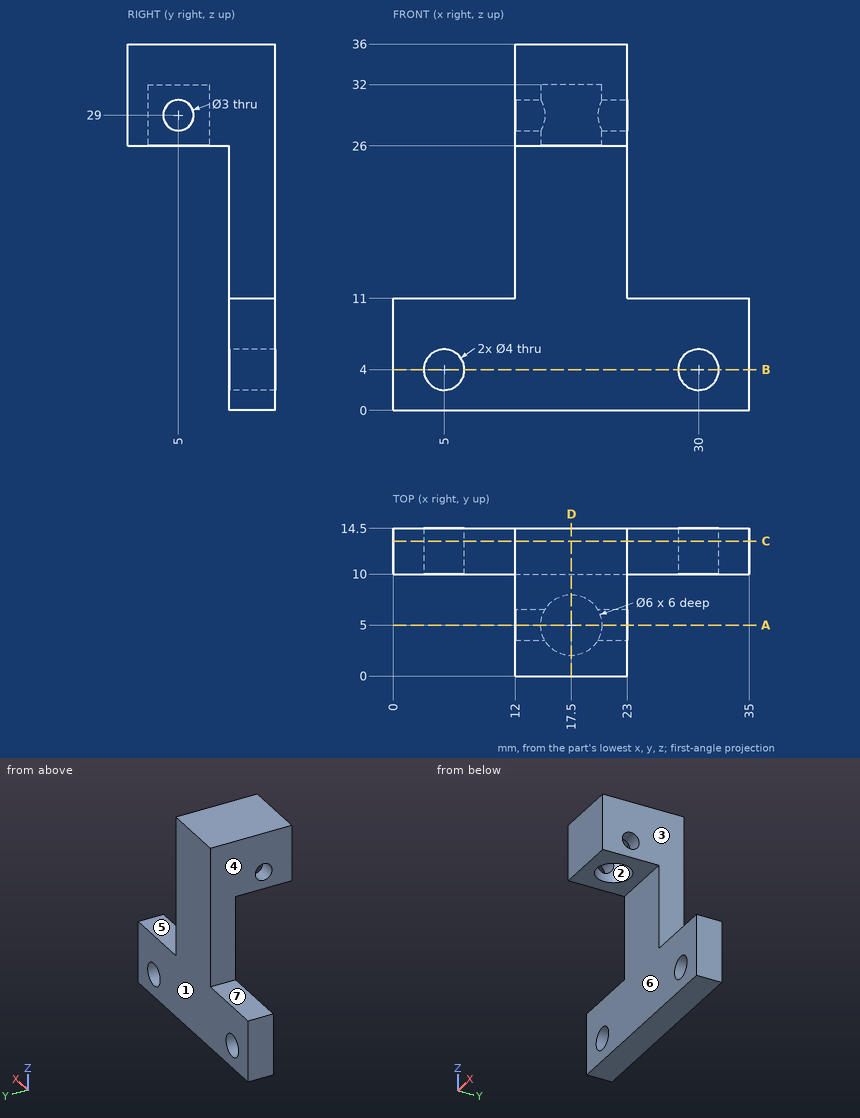
Could you check a few things on this drawing? It's one solid part, dimensions in mm from its lowest x, y, z. A direction names the side the tool comes from. Give positions to 0.01 mm unless a question says otherwise; leave off trailing zeros. Order: outer loops, then holes, each group sorted by start corner. A loop starts at its lowest first (then second) coordinate and runs counter-clockwise, first axis right, second up. Notation, with made-up numbers: (82, -4) -> (118, -4) arc R25 ccw to (118, 12) -> close; hole circle Ø9 at (66.5, -5.5). An arc over 180 degrees is marked (long way). Use CSV: the item, a comma, the result in double quotes. Start each with the question number.
Item 1: Suppose I cut it at B-B (z = 4). List the corners of the cut face in (x, y) for me, and give its area (4 significant figures).
Item 2: On a 3-axis mill with a long thin cutter (end or side, diameter ignored), from which of +Z, -Z, +X, -X, +Y, -Y can I reach the whole of each face in a straight line? I mean the marked faces 5, 6 and 7. Say none if no direction works.
Item 3: Suppose I cut it at D-D (x = 17.5). List the corners of the cut face in (y, z) for me.
Item 4: Suppose I cut it at A-A (y = 5). List the corners of the cut face in (x, z) for me, and give its area (3 significant figures).
Item 5: Thinking about a two-plate mould opening in X: for the marked faces 1, 2, 3 and 4, which applies, pulls with the +X half, pulls with the -X half, needs draft (parallel to the pull), parting line crosses it, or undercut?
Item 6: I'm going to push flat-ended pins straight in: P1, Ø3.5, axis at x = 17.5, y = 5, coming from the -Z side; P2, Ø6, axis at y = 8, z = 15.5, coming from the -X side; P3, Ø4, axis at x = 15.5, z = 10, coming from the -Y side; P4, Ø2.5, axis at x = 5, z = 4, coming from the -Y side. Where does each tip first touch, or does it pass through?
Item 7: Suppose I cut it at C-C (y = 13.25). List the corners of the cut face in (x, z) for me.
Item 8: If I drill on probe 1 along Y at (x, z) = (21.95, 29); probe 2 along Z at (x, y) = (13.75, 5); probe 3 along Y at (x, z) = (17.5, 29.25), over which ranges is the centre line in solid material (lowest first)? Write a range as [from, to].
Answer block:
1,outline,"(0, 10) -> (3, 10) -> (3, 14.5) -> (0, 14.5) -> close; (7, 10) -> (28, 10) -> (28, 14.5) -> (7, 14.5) -> close; (32, 10) -> (35, 10) -> (35, 14.5) -> (32, 14.5) -> close"
1,area,"121.5 mm^2"
2,face 5,"+Z, +X, +Y, -Y"
2,face 6,"-Z, +X, -X, -Y"
2,face 7,"+Z, -X, +Y, -Y"
3,outline,"(0, 26) -> (2, 26) -> (2, 32) -> (8, 32) -> (8, 26) -> (10, 26) -> (10, 0) -> (14.5, 0) -> (14.5, 36) -> (0, 36) -> close"
4,outline,"(12, 26) -> (14.5, 26) -> (14.5, 27.5) -> (12, 27.5) -> close; (12, 30.5) -> (14.5, 30.5) -> (14.5, 32) -> (20.5, 32) -> (20.5, 30.5) -> (23, 30.5) -> (23, 36) -> (12, 36) -> close; (20.5, 26) -> (23, 26) -> (23, 27.5) -> (20.5, 27.5) -> close"
4,area,"59.0 mm^2"
5,face 1,"needs draft"
5,face 2,"undercut"
5,face 3,"pulls with the +X half"
5,face 4,"pulls with the -X half"
6,P1,"stops at z = 32"
6,P2,"stops at x = 12"
6,P3,"stops at y = 10"
6,P4,"passes through"
7,outline,"(0, 0) -> (35, 0) -> (35, 11) -> (23, 11) -> (23, 36) -> (12, 36) -> (12, 11) -> (0, 11) -> close; hole circle Ø4 at (5, 4); hole circle Ø4 at (30, 4)"
8,probe 1,"y = [0, 3.5], [6.5, 14.5]"
8,probe 2,"z = [26, 27.5], [30.5, 36]"
8,probe 3,"y = [0, 2], [8, 14.5]"
